from build123d import *

# Parameters (mm, degrees)
F0_W     = 153.35001
F0_H     = 95.295806
F1_DEPTH = 86.36
F2_SIZE  = 5.08
F3_T     = -2.5


with BuildPart() as f1:
    # F0 (on Front) → F1 (new body)
    with BuildSketch(Plane.XZ):
        with Locations((5.301088, 6.084798)):
            Rectangle(F0_W, F0_H)
    extrude(amount=F1_DEPTH)

    # F2
    f2_edges = [f1.edges().sort_by_distance(p)[0] for p in [
        (5.301088, -86.36, 53.732701),
        (81.976093, -43.18, 53.732701),
        (-71.373917, -43.18, 53.732701),
        (81.976093, -86.36, 6.084798),
        (81.976093, 0, 6.084798),
        (81.976093, -43.18, -41.563105),
    ]]
    chamfer(f2_edges, length=F2_SIZE)

    # F3
    f3_openings = [f1.faces().sort_by_distance(p)[0] for p in [
        (2.761088, -43.18, -41.563105),
    ]]
    offset(amount=F3_T, openings=f3_openings)


solid = f1.part
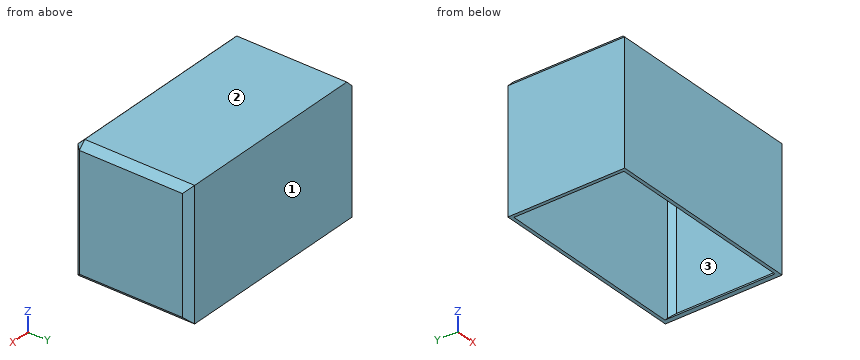
Can you work these out from the model? Positions are in its coordinate system, mm. Face numbers are marked on the shaded views. Give positions to 0.01 mm unless a question says otherwise; leave off trailing zeros. Loops run counter-clockwise (first coordinate to the right, second up) from the corner with the lowest first, then second, coordinate; pieces in that order, holes last. Notation, with made-up numbers: (4.25, 44) - (51.25, 44) arc R24 ccw to (51.25, 65) - close; hole circle Ø3 at (-19.75, 62.25). An arc over 180 degrees is marked (long way). Answer as a JSON object with one key per item and string values.
Q1. Imagine slicing it at C-C on z = 7.5. Write out the boundary of the cut face in (x, y), plus the area to 3 significant figures.
Geometry says:
{"outline": "(-71.37, -86.36) - (76.9, -86.36) - (81.98, -81.28) - (81.98, -5.08) - (76.9, 0) - (-71.37, 0) - close; hole (-68.87, -83.86) - (75.86, -83.86) - (79.48, -80.24) - (79.48, -6.12) - (75.86, -2.5) - (-68.87, -2.5) - close", "area": "1,160 mm²"}
Q2. Will this pin go through, and if not, where does the flat tip stop? P1, Ø8, axis at x = 21, y = -19, coming from the -Z side.
Geometry says:
{"P1": "z = 51.23"}
Q3. Imagine slicing it at A-A on y = -73.5. Write out the boundary of the cut face in (x, z), plus the area to 3 significant figures.
Geometry says:
{"outline": "(-71.37, -41.56) - (-68.87, -41.56) - (-68.87, 47.62) - (-65.26, 51.23) - (75.86, 51.23) - (79.48, 47.62) - (79.48, -35.45) - (73.36, -41.56) - (76.9, -41.56) - (81.98, -36.48) - (81.98, 48.65) - (76.9, 53.73) - (-66.29, 53.73) - (-71.37, 48.65) - close", "area": "840 mm²"}
Q4. Imagine slicing it at B-B on x = 28. Write out the boundary of the cut face in (y, z).
Geometry says:
{"outline": "(-86.36, -41.56) - (-83.86, -41.56) - (-83.86, 47.62) - (-80.24, 51.23) - (-2.5, 51.23) - (-2.5, -41.56) - (0, -41.56) - (0, 53.73) - (-81.28, 53.73) - (-86.36, 48.65) - close"}
Q5. If we mould it in two halves opening along Z, with no side actions, what happens to the marked faces 1, 2 and 3? For each: pulls with the +Z half, pulls with the -Z half, needs draft (parallel to the pull), parting line crosses it, or undercut.
Geometry says:
{"face 1": "needs draft", "face 2": "pulls with the +Z half", "face 3": "undercut"}
Q6. If I drill on L1, parallel to Y at x = -30.5, z = -4; L2, parallel to X at y = -26, z = 30.5; L3, parallel to Z at x = 2.5, y = -39, over which ranges is the centre line in solid material (lowest first)?
Geometry says:
{"L1": "-86.36 to -83.86, -2.5 to 0", "L2": "-71.37 to -68.87, 79.48 to 81.98", "L3": "51.23 to 53.73"}
